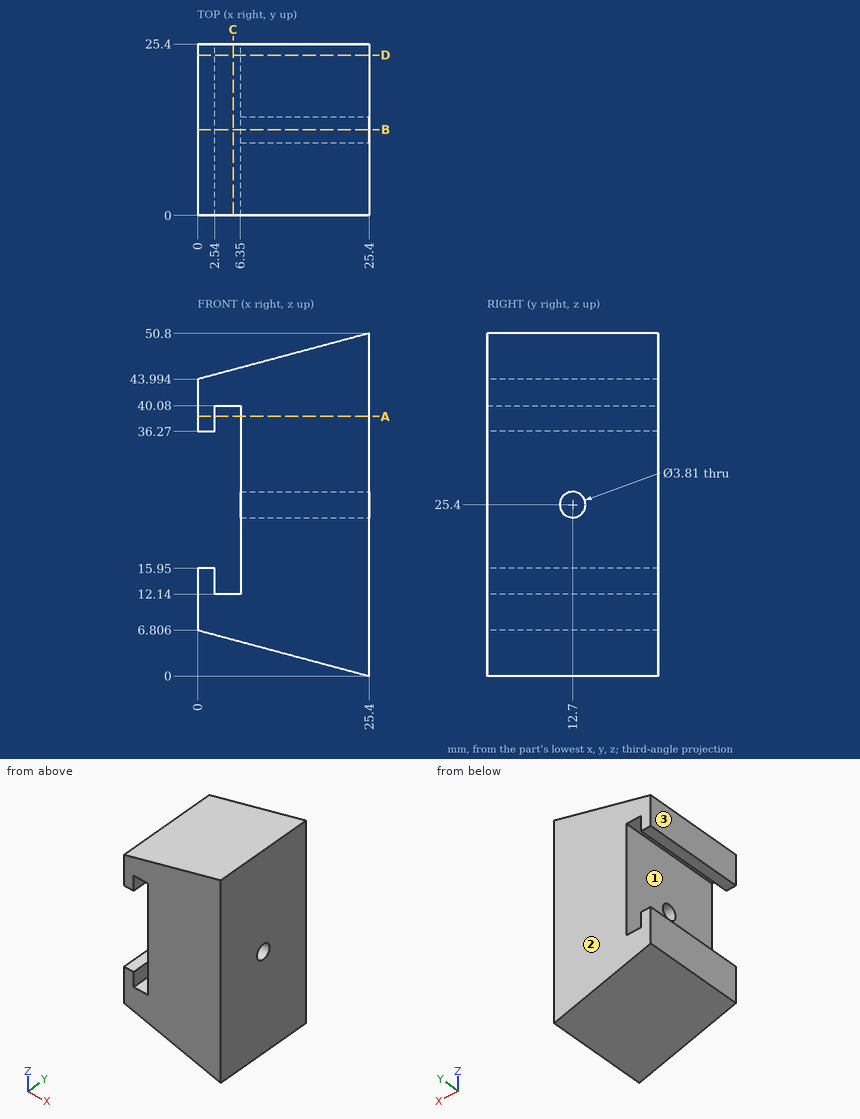
Source: three-view drawing plus pictorial views. Frame: mm from the lowest corner of the part. Give positions to 0.01 mm unless a question says otherwise; leave off trailing zeros. Order: outer loops, then holes, each group sorted by start corner. A loop starts at its lowest first (then second) coordinate and runs counter-clockwise, first axis right, second up. Notation, with made-up numbers: (63, 71) - (77, 71) arc R21 ccw to (77, 109) - close; hole circle Ø4 at (68, 88). An arc over 180 degrees is marked (long way). Answer as a JSON object with one key per item and string values. Group by question number.
Q1. Line query: probe 1 along X at (y, z) = (15.25, 14); probe 2 along X at (y, z) = (14.75, 21); probe 3 along Z at (x, y) = (4.5, 16). Output: solid intervals per line, ascending.
Q2. Cut plane D-D, the plane y = 23.75. Output: boundary loops of the cut face in (x, z).
Q3. First-contact query: pin 1 Ø3 at (x, y) = (3.5, 21) entering from -Z; pin 2 Ø1 at (y, z) = (21.5, 25) entering from -X; pin 3 Ø1.5 at (x, y) = (15, 16.5) entering from -Z. Flat tips, straight axial feed; report the tip coordinate or a pass-through.
Q4. Mould query, pull axis X, two halves, no side actions, for the marked faces 1, 2 and 3. Classes: pulls with the +X half, pulls with the -X half, needs draft (parallel to the pull), parting line crosses it, or undercut.
Q5. Cut plane B-B, the plane y = 12.7. Output: boundary loops of the cut face in (x, z) (3 decimals), then the cut area to 3 significant figures.
Q6. Cut plane A-A, the plane z = 38.5. Output: boundary loops of the cut face in (x, y), then the cut area to 3 significant figures.
Q7. Cut plane C-C, the plane x = 5.25. Output: boundary loops of the cut face in (y, z), then the cut area to 3 significant figures.
Results:
{
 "1": {"probe 1": "0 to 2.54, 6.35 to 25.4", "probe 2": "6.35 to 25.4", "probe 3": "5.6 to 12.14, 40.08 to 45.2"},
 "2": {"outline": "(0, 6.81) - (25.4, 0) - (25.4, 50.8) - (0, 43.99) - (0, 36.27) - (2.54, 36.27) - (2.54, 40.08) - (6.35, 40.08) - (6.35, 12.14) - (2.54, 12.14) - (2.54, 15.95) - (0, 15.95) - close"},
 "3": {"pin 1": "z = 5.47", "pin 2": "x = 6.35", "pin 3": "z = 2.59"},
 "4": {"face 1": "undercut", "face 2": "needs draft", "face 3": "pulls with the -X half"},
 "5": {"outline": "(0, 6.806) - (25.4, 0) - (25.4, 23.495) - (6.35, 23.495) - (6.35, 12.14) - (2.54, 12.14) - (2.54, 15.95) - (0, 15.95) - close; (0, 36.27) - (2.54, 36.27) - (2.54, 40.08) - (6.35, 40.08) - (6.35, 27.305) - (25.4, 27.305) - (25.4, 50.8) - (0, 43.994) - close", "area": "887 mm^2"},
 "6": {"outline": "(0, 0) - (2.54, 0) - (2.54, 25.4) - (0, 25.4) - close; (6.35, 0) - (25.4, 0) - (25.4, 25.4) - (6.35, 25.4) - close", "area": "548 mm^2"},
 "7": {"outline": "(0, 5.4) - (25.4, 5.4) - (25.4, 12.14) - (0, 12.14) - close; (0, 40.08) - (25.4, 40.08) - (25.4, 45.4) - (0, 45.4) - close", "area": "306 mm^2"}
}
